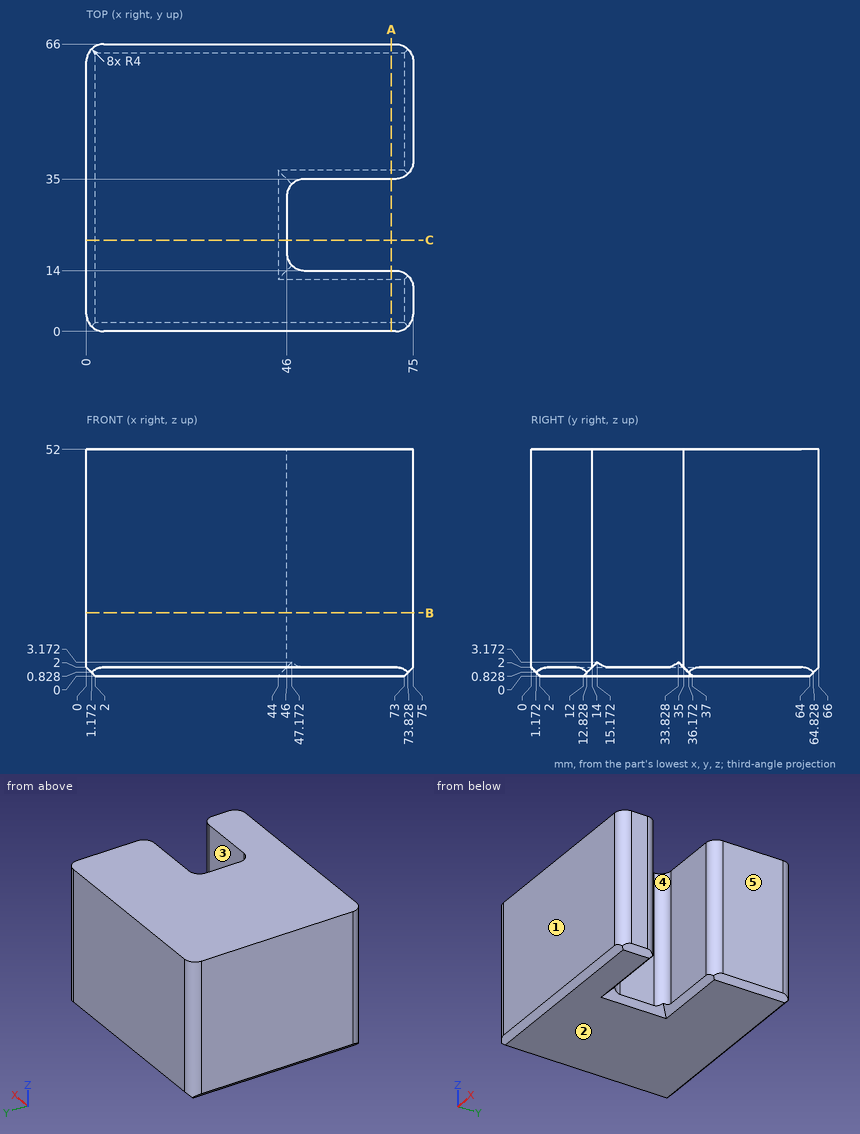
Verification items for this drawing (mm, ordinates from the low corner). A direction names the side the tool comes from. Round coordinates to 2 decimals unless told otherwise and drop trailing zeros. Write each loop counter-clockwise with the first axis right and the second up, starting at its lowest first coordinate (ties: lowest second). Pieces come first, ordered by that corner, then holes. Notation, with made-up numbers: (23.5, 8) - (73.5, 8) arc R7 cw to (73.5, 16) - close; hole circle Ø7 at (-36, -1). An arc over 180 degrees is marked (long way). Answer as a JSON object with one key per item and string values. Group by question number.
Q1. Mould release check, pull along Y, two halves, no side actions. Record for the marked faces 1, 2 and 3: released by +Y, released by -Y, zero draft, split by the parting line, or undercut.
Q2. Thickness scan on line 1 (Y direction, x = 64.5, z = 27.5); line 2 (X direction, y = 30.5, z = 36); line 3 (Y direction, x = 49, z = 40). Record the ranges inside material, lowest first.
Q3. Section check C-C, the plane y = 21. Enter the section's corners in (x, z), plus the area to 3 significant figures.
Q4. Go/stop test with a flat-tipped pin: pin 1 Ø10.5 at (y, z) = (26.5, 30) entering from +X. Record where the tip stops, or that it passes through.
Q5. Tool access check on the marked faces 4 and 5. Record the directions out of +Z, -Z, +X, -X, +Y, -Y that give a thin tool (end or side, any length) a straight path to the whole face; none if there is none.
Q6. Section check B-B, the plane z = 14.5. Enter the section's corners in (x, y).
Q7. Section check A-A, the plane x = 70. Enter the section's corners in (y, z), plus the area to 3 significant figures.
Found:
{
 "1": {"face 1": "released by -Y", "face 2": "zero draft", "face 3": "undercut"},
 "2": {"line 1": "y = 0 to 14, 35 to 66", "line 2": "x = 0 to 46", "line 3": "y = 0 to 14.13, 34.87 to 66"},
 "3": {"outline": "(0, 2) - (2, 0) - (44, 0) - (46, 2) - (46, 52) - (0, 52) - close", "area": "2,390 mm^2"},
 "4": {"pin 1": "stops at x = 46.07"},
 "5": {"face 4": "+Z, -Z, +X", "face 5": "+Z, -Z, +X, +Y, -Y"},
 "6": {"outline": "(0, 4) arc R4 ccw to (4, 0) - (71, 0) arc R4 ccw to (75, 4) - (75, 10) arc R4 ccw to (71, 14) - (50, 14) arc R4 cw to (46, 18) - (46, 31) arc R4 cw to (50, 35) - (71, 35) arc R4 ccw to (75, 39) - (75, 62) arc R4 ccw to (71, 66) - (4, 66) arc R4 ccw to (0, 62) - close"},
 "7": {"outline": "(0, 2) - (2, 0) - (12, 0) - (14, 2) - (14, 52) - (0, 52) - close; (35, 2) - (37, 0) - (64, 0) - (66, 2) - (66, 52) - (35, 52) - close", "area": "2,330 mm^2"}
}
